from build123d import *

# Parameters (mm, degrees)
SKETCH1_W           = 27
SKETCH1_H           = 175
BOSS_EXTRUDE1_DEPTH = 200
SKETCH2_W           = 20
SKETCH2_H           = 30
SKETCH2_R           = 3.071880825
BOSS_EXTRUDE2_DEPTH = 6


with BuildPart() as part:
    # Sketch1 → Boss-Extrude1 (new body)
    with BuildSketch(Plane(origin=(0, 0, 0), x_dir=(1, 0, 0), z_dir=(0, 1, 0))):
        Rectangle(SKETCH1_W, SKETCH1_H)
    extrude(amount=BOSS_EXTRUDE1_DEPTH)

    # Sketch2 → Boss-Extrude2 (add)
    with BuildSketch(Plane(origin=(0, 200, 0), x_dir=(1, 0, 0), z_dir=(0, 1, 0))):
        with Locations((0, -69)):
            Rectangle(SKETCH2_W, SKETCH2_H)
        with Locations((0, -72.5)):
            Circle(SKETCH2_R, mode=Mode.SUBTRACT)
        with Locations((0, 69)):
            Rectangle(SKETCH2_W, SKETCH2_H)
        with Locations((0, 72.5)):
            Circle(SKETCH2_R, mode=Mode.SUBTRACT)
    extrude(amount=BOSS_EXTRUDE2_DEPTH)


solid = part.part
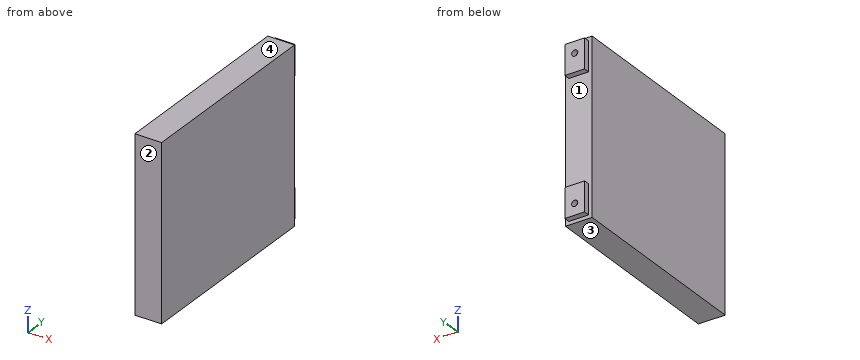
Design review of the part built by this model. Coordinates are the model's own, in mm. Face numbers are marked on the shaded views. Give positions to 0.01 mm unless a question says otherwise; leave off trailing zeros. Order: outer loops, then holes, each group sorted by start corner. A loop starts at its lowest first (then second) coordinate and runs counter-clockwise, first axis right, second up.
1. To check wall thickness, follow L1, parallel to Z at x = 0, y = 203.8; L2, parallel to X at y = 203.3, z = 72.5; L3, parallel to X at y = 202, z = 72. State the ranges of each line that lie inside material, in increasing order.
Solution:
L1: z = -84 to -75.57, -69.43 to -54, 54 to 69.43, 75.57 to 84
L2: x = -10 to -3.07, 3.07 to 10
L3: x = -10 to -3.03, 3.03 to 10
2. Add section A-A, the plane x = 0. State the section outline as (y, z) points.
Solution:
outline: (0, -87.5) - (200, -87.5) - (200, -84) - (206, -84) - (206, -75.57) - (200, -75.57) - (200, -69.43) - (206, -69.43) - (206, -54) - (200, -54) - (200, 54) - (206, 54) - (206, 69.43) - (200, 69.43) - (200, 75.57) - (206, 75.57) - (206, 84) - (200, 84) - (200, 87.5) - (0, 87.5) - close
3. For pin 1 Ø5 at (x, z) = (0, -72.5) entering from +Y; pin 2 Ø6.5 at (x, y) = (-1, 203.5) entering from -Z; pin 3 Ø3 at (y, z) = (204.5, 63.5) entering from +X, all flat-tipped, find the tip position at first contact; note any pin that passes through.
Solution:
pin 1: stops at y = 200
pin 2: stops at z = -84
pin 3: stops at x = 10
4. Mouldability with a two-part tool opening along Z and no side actions: class the marked faces 1, 2, 3 and 4 as +Z half, -Z half, draft (parallel to the pull), parting line (faces both ways), or undercut.
Solution:
face 1: undercut
face 2: draft
face 3: -Z half
face 4: +Z half
5. Add section B-B, the plane z = -5.5. State the section outline as (x, y) points, then the cut area to 3 significant figures.
Solution:
outline: (-13.5, 0) - (13.5, 0) - (13.5, 200) - (-13.5, 200) - close
area: 5,400 mm2
